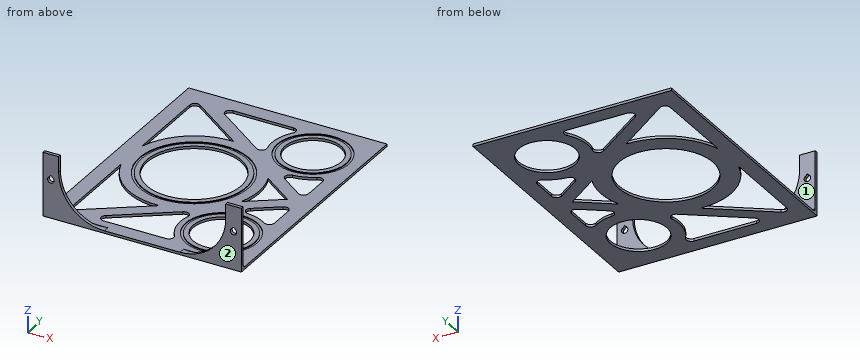
Autodesk Fusion 360 part; units mm, degrees
sketch "Sketch1" plane through (0, 0, 0) normal (0, 0, 1) x (1, 0, 0)
  line L0 (-74.0678, 23.5735) -> (-61.5678, 23.5735)
  line L1 (-61.5678, 23.5735) -> (-61.5678, 226.7735)
  line L2 (-61.5678, 226.7735) -> (-74.0678, 226.7735)
  line L3 (-74.0678, 226.7735) -> (-74.0678, 23.5735)
  line L4 (71.9322, 23.5735) -> (84.4322, 23.5735)
  line L5 (84.4322, 23.5735) -> (84.4322, 226.7735)
  line L6 (84.4322, 226.7735) -> (71.9322, 226.7735)
  line L7 (71.9322, 226.7735) -> (71.9322, 23.5735)
  line L8 (-32, 23.5735) -> (47, 23.5735) construction
  circle A0 centre (-67.8178, 5.0413) radius 2.55 construction
  circle A1 centre (78.1822, 4.9635) radius 2.55 construction
  line L9 (-74.0678, 26.0735) -> (-61.5678, 26.0735)
  line L10 (-61.5678, 26.0735) -> (-61.5678, 23.5735)
  line L11 (-61.5678, 23.5735) -> (-74.0678, 23.5735)
  line L12 (-74.0678, 23.5735) -> (-74.0678, 26.0735)
  line L13 (71.9322, 26.0735) -> (84.4322, 26.0735)
  line L14 (84.4322, 26.0735) -> (84.4322, 23.5735)
  line L15 (84.4322, 23.5735) -> (71.9322, 23.5735)
  line L16 (71.9322, 23.5735) -> (71.9322, 26.0735)
  line L17 (55.3253, 131.4235) -> (71.9322, 131.4235) construction
  line L18 (71.9322, 131.4235) -> (71.9322, 118.9235) construction
  line L19 (71.9322, 118.9235) -> (55.3253, 118.9235) construction
  line L20 (55.3253, 118.9235) -> (55.3253, 131.4235) construction
  line L21 (-61.5678, 23.5735) -> (71.9322, 118.9235)
  line L22 (71.9322, 131.4235) -> (-61.5678, 36.0735)
  line L23 (71.9322, 131.4235) -> (-61.5678, 226.7735)
  line L24 (71.9322, 118.9235) -> (-61.5678, 214.2735)
  line L25 (-61.5678, 23.5735) -> (71.9322, 23.5735)
  line L26 (67.9766, 35.4311) -> (-44.9659, 35.4311)
  circle A2 centre (46.9322, 61.3246) radius 22.5
  circle A3 centre (46.9322, 61.3246) radius 32.817
  circle A4 centre (-11.5678, 125.1735) radius 37.5
  circle A5 centre (-11.5678, 125.1735) radius 51.943
  line L27 (-61.5678, 226.7735) -> (71.9322, 226.7735)
  line L28 (71.9322, 214.2735) -> (-44.0665, 214.2735)
  line L29 (84.4322, 125.1735) -> (-74.0678, 125.1735) construction
  circle A6 centre (46.9322, 189.0223) radius 32.817
  circle A7 centre (46.9322, 189.0223) radius 22.5
  point P0 (-67.8178, 23.5735)
  point P1 (78.1822, 23.5735)
  point P2 (71.9322, 125.1735)
  point P3 (71.9322, 125.1735)
  dimension "d1" = 12.5
  dimension "d2" = 12.5
  dimension "d3" = 5.1
  dimension "d4" = 5.1
  dimension "d7" = 146
  dimension "d8" = 203.2
  dimension "d9" = 2.5
  dimension "d10" = 2.5
  dimension "d16" = 12.5
  dimension "d17" = 12.5
  dimension "d18" = 12.5
  dimension "d19" = 12.5
  dimension "d20" = 10.317
  dimension "d21" = 14.443
  dimension "d24" = 12.5
  dimension "d27" = 45
  dimension "d28" = 25
  dimension "d29" = 50
  dimension "d30" = 75
extrude "Extrude1" add sketch "Sketch1" along normal blind 50.8 contours L0 L1 L3 L9 L10 L11 L12 | L4 L5 L7 L13 L14 L15 L16 makes body 1 at (-69.9011, 26.0735, 16.9333) makes body 2 at (76.0989, 23.5735, 16.9333)
ref_plane "WorkPlane1" through (5.1822, 24.8235, 25.4) normal (1, 0, 0) x (0, 1, 0)
sketch "Sketch2" plane through (0, 23.5735, 0) normal (0, -1, 0) x (1, 0, 0)
  line L0 (-74.0678, 0) -> (-61.5678, 0)
  line L1 (-61.5678, 0) -> (-61.5678, 50.8)
  line L2 (-61.5678, 50.8) -> (-74.0678, 50.8)
  line L3 (-74.0678, 50.8) -> (-74.0678, 0)
  circle A0 centre (-67.8178, 30.5) radius 2.55
  line L4 (-74.0678, 0) -> (-61.5678, 0)
  line L5 (5.1822, 55.88) -> (5.1822, -5.08)
  circle A1 centre (78.1822, 30.5) radius 2.55
  line L6 (-69.5607, 32.3613) -> (-67.79, 34.0194)
  line L7 (-67.79, 34.0194) -> (-66.0457, 32.3336)
  line L8 (79.9252, 32.3613) -> (78.1545, 34.0194)
  line L9 (78.1545, 34.0194) -> (76.4101, 32.3336)
  point P0 (-67.8178, 50.8)
  dimension "d13" = 5.1
  dimension "d14" = 30.5
extrude "Extrude2" cut sketch "Sketch2" against normal through all contours A0 | A0 L6 L7 | A1 | A1 L8 L9 bodies 1 2
extrude "Extrude3" add sketch "Sketch1" along normal blind 2 contours L1 L10 L21 L22 L24 A3 A5 | L7 L16 L21 L25 L26 A3 | L1 L2 L3 L9 A5 | L21 A3 | L7 L21 L26 A3 | L26 A3 | L5 L6 L7 L13 A3 A6 | L1 L22 L23 L24 A5 A6 | L7 L23 L27 L28 A6 | L1 A5 | L1 L22 L24 A5 | L22 A5 | L7 A3 | L7 L22 L24 | L24 A5 | L7 L23 L28 A6 | L23 A6 | L28 A6 | L7 L28 A6 | L7 A6 bodies 1 2
fillet "Fillet2" radius 4 14 edges at (-61.5678, 36.0735, 1) (23.6038, 84.4057, 1) (26.7709, 35.4311, 1) (32.6668, 90.8788, 1) (71.9322, 118.9235, 1) (71.9322, 131.4235, 1) (32.6668, 159.4681, 1) (71.9322, 167.7631, 1) (-44.0665, 214.2735, 1) (23.6038, 165.9412, 1) (25.972, 214.2735, 1) (-61.5678, 214.2735, 1) (71.9322, 82.5838, 1) (-44.9659, 35.4311, 1) on bodies 1
sketch "Sketch3" plane through (0, 0, 2) normal (0, 0, 1) x (-1, 0, 0)
  line L0 (61.5678, -23.5735) -> (-71.9322, -23.5735)
  line L1 (-84.4322, -26.0735) -> (-84.4322, -226.7735)
  line L2 (-84.4322, -226.7735) -> (74.0678, -226.7735)
  line L3 (74.0678, -226.7735) -> (74.0678, -26.0735)
  line L4 (-36.8514, -143.9793) -> (-63.1816, -125.1735)
  line L5 (-63.1816, -125.1735) -> (-36.8514, -106.3676)
  arc A0 (-36.8514, -106.3676) -> (-36.8514, -143.9793) centre (11.5678, -125.1735) ccw
  line L6 (-47.2589, -101.301) -> (-65.6074, -114.4061)
  arc A1 (-71.9322, -111.151) -> (-65.6074, -114.4061) centre (-67.9322, -111.151) ccw
  line L7 (-71.9322, -111.151) -> (-71.9322, -91.5651)
  arc A2 (-65.6507, -88.2796) -> (-71.9322, -91.5651) centre (-67.9322, -91.5651) ccw
  arc A3 (-65.6507, -88.2796) -> (-49.2957, -94.0564) centre (-46.9322, -61.3246) ccw
  arc A4 (-47.2589, -101.301) -> (-49.2957, -94.0564) centre (-49.5838, -98.046) ccw
  circle A5 centre (11.5678, -125.1735) radius 37.5
  circle A6 centre (-46.9322, -189.0223) radius 22.5
  line L8 (55.2429, -209.7561) -> (9.4856, -177.0747)
  arc A7 (9.4856, -177.0747) -> (61.5678, -139.2473) centre (11.5678, -125.1735) ccw
  line L9 (61.5678, -139.2473) -> (61.5678, -206.501)
  arc A8 (55.2429, -209.7561) -> (61.5678, -206.501) centre (57.5678, -206.501) ccw
  circle A9 centre (-46.9322, -61.3246) radius 22.5
  arc A10 (-49.2957, -156.2905) -> (-65.6507, -162.0673) centre (-46.9322, -189.0223) ccw
  arc A11 (-71.9322, -158.7818) -> (-65.6507, -162.0673) centre (-67.9322, -158.7818) ccw
  line L10 (-71.9322, -158.7818) -> (-71.9322, -139.1959)
  arc A12 (-65.6074, -135.9409) -> (-71.9322, -139.1959) centre (-67.9322, -139.1959) ccw
  line L11 (-65.6074, -135.9409) -> (-47.2589, -149.0459)
  arc A13 (-49.2957, -156.2905) -> (-47.2589, -149.0459) centre (-49.5838, -152.3009) ccw
  line L12 (34.8081, -42.6861) -> (-9.0117, -73.9836)
  arc A14 (-15.2038, -69.7068) -> (-9.0117, -73.9836) centre (-11.3365, -70.7285) ccw
  arc A15 (-15.2038, -69.7068) -> (-20.5481, -41.8097) centre (-46.9322, -61.3246) ccw
  arc A16 (-17.3322, -35.4311) -> (-20.5481, -41.8097) centre (-17.3322, -39.4311) ccw
  line L13 (-17.3322, -35.4311) -> (32.4832, -35.4311)
  arc A17 (34.8081, -42.6861) -> (32.4832, -35.4311) centre (32.4832, -39.4311) ccw
  line L14 (61.5678, -43.8459) -> (61.5678, -111.0996)
  arc A18 (61.5678, -111.0996) -> (9.4856, -73.2722) centre (11.5678, -125.1735) ccw
  line L15 (9.4856, -73.2722) -> (55.2429, -40.5909)
  arc A19 (61.5678, -43.8459) -> (55.2429, -40.5909) centre (57.5678, -43.8459) ccw
  line L16 (31.5838, -214.2735) -> (-16.8677, -214.2735)
  arc A20 (-20.1341, -207.9646) -> (-16.8677, -214.2735) centre (-16.8677, -210.2735) ccw
  arc A21 (-20.1341, -207.9646) -> (-15.2038, -180.6401) centre (-46.9322, -189.0223) ccw
  arc A22 (-9.0117, -176.3633) -> (-15.2038, -180.6401) centre (-11.3365, -179.6184) ccw
  line L17 (-9.0117, -176.3633) -> (33.9087, -207.0184)
  arc A23 (31.5838, -214.2735) -> (33.9087, -207.0184) centre (31.5838, -210.2735) ccw
  circle A24 centre (-46.9322, -61.3246) radius 26.5
  circle A25 centre (-46.9322, -61.3246) radius 28.5
  circle A26 centre (11.5678, -125.1735) radius 41.5
  circle A27 centre (11.5678, -125.1735) radius 43.5
  circle A28 centre (-46.9322, -189.0223) radius 26.5
  circle A29 centre (-46.9322, -189.0223) radius 28.5
  line L18 (74.0678, -26.0735) -> (61.5678, -26.0735)
  line L19 (61.5678, -26.0735) -> (61.5678, -23.5735)
  line L20 (-71.9322, -23.5735) -> (-71.9322, -26.0735)
  line L21 (-71.9322, -26.0735) -> (-84.4322, -26.0735)
  dimension "d31" = 4
  dimension "d32" = 6
  dimension "d33" = 4
  dimension "d34" = 6
  dimension "d35" = 4
  dimension "d36" = 6
extrude "Extrude4" cut sketch "Sketch3" against normal blind 0.5 contours A25 | A27 | A29 bodies 1
fillet "Fillet3" radius 36.5 2 edges at (-61.5678, 24.8235, 2) (71.9322, 24.8235, 2) on bodies 1
fillet "Fillet4" radius 2.5 2 edges at (59.9322, 26.0735, 2) (-49.5678, 26.0735, 2) on bodies 1
Here's how the part is built. I have some questions about the finished solid (model axes, mm). Face numbers are marked on the shaded views. A direction names the side the tool comes from. Coordinates: 2 decimals unless noted, no trailing zeros. Order: outer loops, then holes, each group sorted by start corner. A loop starts at its lowest first (then second) coordinate and runs counter-clockwise, first axis right, second up. Notation, with made-up numbers: M 38,79 L 56,79 A21 cw 56,112 Z; hole C -37.5,76.5 d7. An arc over 180 degrees is marked long. Answer as a JSON object with one key per item and string values. Group by question number.
(1) For pin 1 (16 mm diameter, centred on x = 45.5, y = 51.5, fed in from +Z), with a flat end and sliding along its axis, tell me the tip position at first contact or that it passes through.
(2) Suppose I cut it at D-D, the plane x = 2. Please give me the cut outline in (y, z), then the cut area to 3 significant figures.
(3) Suppose I cut it at C-C, the plane x = -16. State how many separate pieces and enclosed holes the cut face has, then the cut area to 3 significant figures.
(4) Which directions (+Z, -Z, +X, -X, +Y, -Y) give clear straight access to the entire face, cutting with the end or side of a thin tool? Please do the marked faces 1 and 2.
(5) I need wall thicknesses on probe 1 along Z at (x, y) = (32.5, 167.5); probe 2 along Z at (x, y) = (74.5, 184); probe 3 along Y at (x, z) = (-67, 47). Which ranges of each line are inside material? Lowest first, please.
(6) Suppose I cut it at B-B, the plane y = 64. Please give me the cut outline in (x, z), then the cut area to 3 significant figures.
(7) Suppose I cut it at A-A, the plane z = 42.5. Please give me the cut outline in (x, y), then the cut area to 3 significant figures.
Values found:
{
 "1": {"pin 1": "passes through"},
 "2": {"outline": "M 23.57,0 L 35.43,0 L 35.43,2 L 23.57,2 Z; M 68.98,0 L 90.21,0 L 90.21,2 L 85.95,2 L 85.95,1.5 L 83.84,1.5 L 83.84,2 L 68.98,2 Z; M 160.13,0 L 181.37,0 L 181.37,2 L 166.5,2 L 166.5,1.5 L 164.39,1.5 L 164.39,2 L 160.13,2 Z; M 214.27,0 L 226.77,0 L 226.77,2 L 214.27,2 Z", "area": "132 mm^2"},
 "3": {"separate pieces": "6", "enclosed holes": "0", "area": "155 mm^2"},
 "4": {"face 1": "+Z, +X, -X, +Y", "face 2": "+Z, -Z, +X, -X, -Y"},
 "5": {"probe 1": "z = 0 to 2", "probe 2": "z = 0 to 1.5", "probe 3": "y = 23.57 to 26.07"},
 "6": {"outline": "M -74.07,0 L -61.57,0 L -61.57,2 L -74.07,2 Z; M -22.47,0 L -4.97,0 L -4.97,2 L -22.47,2 Z; M 14.22,0 L 24.59,0 L 24.59,2 L 20.57,2 L 20.57,1.5 L 18.56,1.5 L 18.56,2 L 14.22,2 Z; M 69.27,0 L 84.43,0 L 84.43,2 L 75.31,2 L 75.31,1.5 L 73.3,1.5 L 73.3,2 L 69.27,2 Z", "area": "109 mm^2"},
 "7": {"outline": "M -74.07,23.57 L -61.57,23.57 L -61.57,26.07 L -74.07,26.07 Z; M 71.93,23.57 L 84.43,23.57 L 84.43,26.07 L 71.93,26.07 Z", "area": "62.5 mm^2"}
}
